Geometry check sheet. Reference: the model listing, model coordinates, mm. Face numbers are marked on the shaded views. Coordinates: 2 decimals unless noted, no trailing zeros. Loops run counter-clockwise (first coordinate to the right, second up) from the corner with the lowest first, then second, coordinate; pieces in that order, holes last. Notation, with made-up numbers: M 72,-1 L 92,-1 A22 ccw 92,10 Z; hole C 21.5,68.25 d9. An arc over 180 degrees is marked long. Use CSV: the item, a comma, the result in double quotes.
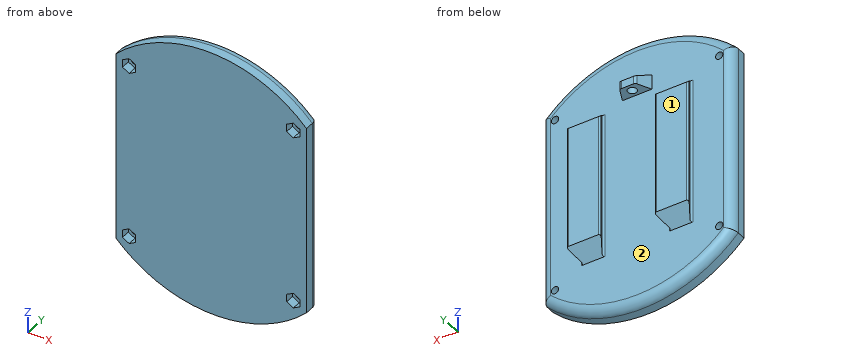
```python
from build123d import *

# Parameters (mm, degrees)
EXTRUDE_1_DEPTH     = 6
CUT_EXTRUDE_1_DEPTH = 3
SKETCH_4_R          = 1.25
CUT_EXTRUDE_3_DEPTH = 57.402570863
EXTRUDE_2_DEPTH     = 25
DRAFT_1_ANGLE       = 40
FILLET_1_R          = 0.5
SKETCH_6_W          = 10
SKETCH_6_H          = 5
EXTRUDE_3_DEPTH     = 5
DRAFT_3_ANGLE       = 25
FILLET_2_R          = 1
SKETCH_7_R          = 1.5
CUT_EXTRUDE_4_DEPTH = 5
SKETCH_8_R          = 2
SKETCH_8_R_2        = 1.5
CUT_EXTRUDE_5_DEPTH = 2
DRAFT_START         = 31.990712649
DRAFT_5_DEPTH       = 3.009287351
FILLET_3_R          = 3


with BuildPart() as part:
    # Эскиз1 → Бобышка-Вытянуть1 (new body)
    with BuildSketch(Plane(origin=(0, 0, 0), x_dir=(1, 0, 0), z_dir=(0, 1, 0))):
        with BuildLine():
            Line((-32.5, -32.5), (-32.5, 32.5))
            ThreePointArc((-32.5, 32.5), (0, 46), (32.5, 32.5))
            Line((32.5, 32.5), (32.5, -32.5))
            ThreePointArc((32.5, -32.5), (0, -46), (-32.5, -32.5))
        make_face()
    extrude(amount=EXTRUDE_1_DEPTH)

    # Эскиз2 → Вырез-Вытянуть1 (cut)
    with BuildSketch(Plane.XZ):
        Polygon((28, -32.598076211), (30.25, -31.299038106), (30.25, -28.700961894), (28, -27.401923789), (25.75, -28.700961894), (25.75, -31.299038106), align=None)
        Polygon((25.75, 31.299038106), (25.75, 28.700961894), (28, 27.401923789), (30.25, 28.700961894), (30.25, 31.299038106), (28, 32.598076211), align=None)
        Polygon((-28, 27.401923789), (-25.75, 28.700961894), (-25.75, 31.299038106), (-28, 32.598076211), (-30.25, 31.299038106), (-30.25, 28.700961894), align=None)
        Polygon((-28, -32.598076211), (-25.75, -31.299038106), (-25.75, -28.700961894), (-28, -27.401923789), (-30.25, -28.700961894), (-30.25, -31.299038106), align=None)
    extrude(amount=-CUT_EXTRUDE_1_DEPTH, mode=Mode.SUBTRACT)

    # Эскиз4 → Вырез-Вытянуть3 (cut, through all)
    with BuildSketch(Plane.XZ.offset(-3)):
        with Locations(Location((28, 30, 0), (0, 0, 270))):
            Circle(SKETCH_4_R)
        with Locations(Location((-28, 30, 0), (0, 0, 270))):
            Circle(SKETCH_4_R)
        with Locations(Location((-28, -30, 0), (0, 0, 270))):
            Circle(SKETCH_4_R)
        with Locations(Location((28, -30, 0), (0, 0, 270))):
            Circle(SKETCH_4_R)
    extrude(amount=-CUT_EXTRUDE_3_DEPTH, mode=Mode.SUBTRACT)

    # Эскиз5 → Бобышка-Вытянуть2 (add, symmetric)
    with BuildSketch(Plane.XY):
        Polygon((-18.113248654, 6), (-11.886751346, 6), (-9, 11), (-21, 11), align=None)
        Polygon((21, 11), (9, 11), (11.886751346, 6), (18.113248654, 6), align=None)
    extrude(amount=EXTRUDE_2_DEPTH, both=True)

    # Уклон1
    draft_1_faces = [part.faces().sort_by_distance(p)[0] for p in [
        (15, 8.763970206, -25),
        (15, 8.763970206, 25),
        (-15, 8.763970206, -25),
        (-15, 8.763970206, 25),
    ]]
    draft(draft_1_faces, Plane.ZX.offset(6), DRAFT_1_ANGLE)

    # Скругление1
    fillet_1_edges = [part.edges().sort_by_distance(p)[0] for p in [
        (-9, 11, 0),
        (-21, 11, 0),
        (-18.113248654, 6, 0),
        (-11.886751346, 6, 0),
        (11.886751346, 6, 0),
        (18.113248654, 6, 0),
        (21, 11, 0),
        (9, 11, 0),
    ]]
    fillet(fillet_1_edges, radius=FILLET_1_R)

    # Эскиз6 → Бобышка-Вытянуть3 (add)
    with BuildSketch(Plane(origin=(0, 6, 0), x_dir=(1, 0, 0), z_dir=(0, 1, 0))):
        with Locations((0, -30)):
            Rectangle(SKETCH_6_W, SKETCH_6_H)
    extrude(amount=EXTRUDE_3_DEPTH)

    # Уклон3
    draft_3_faces = [part.faces().sort_by_distance(p)[0] for p in [
        (5, 8.5, 30),
        (-5, 8.5, 30),
    ]]
    draft(draft_3_faces, Plane.ZX.offset(6), DRAFT_3_ANGLE)

    # Скругление2
    fillet_2_edges = [part.edges().sort_by_distance(p)[0] for p in [
        (2.668461709, 11, 30),
        (-2.668461709, 11, 30),
    ]]
    fillet(fillet_2_edges, radius=FILLET_2_R)

    # Эскиз7 → Вырез-Вытянуть4 (cut)
    with BuildSketch(Plane.XY.offset(32.5)):
        with Locations((0, 8.5)):
            Circle(SKETCH_7_R)
    extrude(amount=-CUT_EXTRUDE_4_DEPTH, mode=Mode.SUBTRACT)

    # Эскиз8 → Вырез-Вытянуть5 (cut)
    with BuildSketch(Plane.XY.offset(32.5)):
        with Locations((0, 8.5)):
            Circle(SKETCH_8_R)
        with Locations((0, 8.5)):
            Circle(SKETCH_8_R_2, mode=Mode.SUBTRACT)
    extrude(amount=-CUT_EXTRUDE_5_DEPTH, mode=Mode.SUBTRACT)

    # Уклон5: read off the stored shape, not the designer's step
    # Уклон5 outline → Уклон5 (cut)
    with BuildSketch(Plane(origin=(0, 0, 0), x_dir=(1, 0, 0), z_dir=(0, 0.4226182617406999, 0.9063077870366498)).offset(DRAFT_START)):
        with BuildLine():
            Line((-5, -8.297246784), (5, -8.297246784))
            Line((5, -8.297246784), (2.937699235, -3.41742745))
            add(Edge.make_bspline(
                [(2.937699235, -3.41742745), (2.668461709, -2.78035719), (2.031391448, -2.78035719)],
                knots=[2.00712864, 2.00712864, 2.00712864, 3.141592654, 3.141592654, 3.141592654], degree=2, weights=[1, 0.843391446, 1]))
            Line((2.031391448, -2.78035719), (-2.031391448, -2.78035719))
            add(Edge.make_bspline(
                [(-2.031391448, -2.78035719), (-2.668461709, -2.78035719), (-2.937699235, -3.41742745)],
                knots=[0, 0, 0, 1.134464014, 1.134464014, 1.134464014], degree=2, weights=[1, 0.843391446, 1]))
            Line((-2.937699235, -3.41742745), (-5, -8.297246784))
        make_face()
    extrude(amount=DRAFT_5_DEPTH, mode=Mode.SUBTRACT)

    # Скругление3
    fillet_3_edges = [part.edges().sort_by_distance(p)[0] for p in [
        (0, 6, 46),
        (32.5, 6, 0),
        (0, 6, -46),
        (-32.5, 6, 0),
    ]]
    fillet(fillet_3_edges, radius=FILLET_3_R)


solid = part.part
```
1. Section check C-C, the plane y = 8.5. Record the cut outline in (x, z), plus the area to 3 significant figures.
The answers:
outline,"M -19.56,-22.9 L -10.44,-22.9 L -10.44,22.9 L -19.56,22.9 Z; M -3.83,27.5 L -1.5,27.5 L -1.5,30.5 L -2,30.5 L -2,31.33 L -3.83,31.33 Z; M 1.5,27.5 L 3.83,27.5 L 3.83,31.33 L 2,31.33 L 2,30.5 L 1.5,30.5 Z; M 10.44,-22.9 L 19.56,-22.9 L 19.56,22.9 L 10.44,22.9 Z"
area,"852 mm^2"
2. Section check D-D, the plane z = -15. Record the cut outline in (x, y), plus the area to 3 significant figures.
The answers:
outline,"M -32.5,0 L 32.5,0 L 32.5,3 A3 ccw 29.5,6 L 18.98,6 A0.5 cw 18.55,6.75 L 20.57,10.25 A0.5 ccw 20.13,11 L 9.87,11 A0.5 ccw 9.43,10.25 L 11.45,6.75 A0.5 cw 11.02,6 L -11.02,6 A0.5 cw -11.45,6.75 L -9.43,10.25 A0.5 ccw -9.87,11 L -20.13,11 A0.5 ccw -20.57,10.25 L -18.55,6.75 A0.5 cw -18.98,6 L -29.5,6 A3 ccw -32.5,3 Z"
area,"477 mm^2"
3. Thickness scan on line 1 (X direction, y = 3.9, z = -30); line 2 (X direction, y = 4.6, z = -30); line 3 (Y direction, x = -2.5, z = -33). Record the ranges inside material, lowest first. Write a range as [from, to].
The answers:
line 1,"[-32.36, -29.25], [-26.75, 26.75], [29.25, 32.36]"
line 2,"[-32.04, -29.25], [-26.75, 26.75], [29.25, 32.04]"
line 3,"[0, 6]"
4. Release check for a two-part mould opening along X. For the marked faces 1 and 2 record: +X half, -X half, draft (parallel to the pull), parting line (faces both ways), or undercut.
The answers:
face 1,"draft"
face 2,"undercut"
5. Section check B-B, the plane y = 4.5. Record the cut outline in (x, z), plus the area to 4 significant figures.
The answers:
outline,"M -32.1,-32.33 A45.47 ccw 32.1,-32.33 L 32.1,32.33 A45.47 ccw -32.1,32.33 Z; hole C -28,-30 d2.5; hole C -28,30 d2.5; hole C 28,-30 d2.5; hole C 28,30 d2.5"
area,"5,305 mm^2"
6. Section check A-A, the plane z = -30. Record the cut outline in (x, y).
The answers:
outline,"M -32.5,0 L -30.25,0 L -30.25,3 L -29.25,3 L -29.25,6 L -29.5,6 A3 ccw -32.5,3 Z; M -26.75,3 L -25.75,3 L -25.75,0 L 25.75,0 L 25.75,3 L 26.75,3 L 26.75,6 L -26.75,6 Z; M 29.25,3 L 30.25,3 L 30.25,0 L 32.5,0 L 32.5,3 A3 ccw 29.5,6 L 29.25,6 Z"
7. Gauge pin test, flat ends, axial feed: P1, Ø2, axis at x = -2.5, z = 32.5, coming from the +Y side; P2, Ø2, axis at x = -28, z = 30.5, coming from the -Y side; P3, Ø5, axis at x = 17.5, z = 35, coming from the +Y side; P4, Ø2, axis at x = -28, z = -30, coming from the -Y side. Record the tip position at first contact, or that the pin passes through.
The answers:
P1,"y = 8.14"
P2,"y = 3"
P3,"y = 6"
P4,"through"
